from build123d import *

# Parameters (mm, degrees)
F1_DEPTH = 152.4


with BuildPart() as f1:
    # F0 (on Front) → F1 (new body)
    with BuildSketch(Plane.XZ):
        Polygon((-58.954738, 0), (0, 0), (0, 16.688244), (-43.046318, 16.688244), (-43.046318, 30.101229), (-43.046318, 54.935103), (-58.954738, 60.358422), align=None)
    extrude(amount=F1_DEPTH)

    # F1_face (on face) → F2 (revolve)
    with BuildSketch(Plane(origin=(-38.122493, -152.4, 19.839762), x_dir=(1, 0, 0), z_dir=(0, -1, 0))):
        Polygon((-20.832245, 40.51866), (-20.832245, -19.839762), (38.122493, -19.839762), (38.122493, -3.151518), (-4.923825, -3.151518), (-4.923825, 35.095341), align=None)
    revolve(axis=Axis((0, -152.4, 8.344122), (0, 0, -1)))


solid = f1.part
Work out the finished part from the listing and answer in its coordinate system (mm). A direction names the side the tool comes from. Coordinates: 2 decimals unless noted, no trailing zeros. Write each loop counter-clockwise with the first axis right and the second up, starting at its lowest first coordinate (ties: lowest second). Pieces come first, ordered by that corner, then holes.
1. For a pull along X with two mould halves and no side action, classify faces 1 (the conical face through (5.733, -108.733, 55.274)), 2 (the flat face through (-12, -128, 0)), 3 (the flat face through (0, -46, 8)) as +X half, -X half, draft (parallel to the pull), parting line (faces both ways), or undercut.
Results list:
face 1: undercut
face 2: draft
face 3: +X half
2. Flat-ended cylindrical pins translate along their axes: pin 1 (10 mm diameter, centred on x = 38, y = -172, fed in from -Z); pin 2 (10 mm diameter, centred on y = -85, z = 54, fed in from +X); pin 3 (4 mm diameter, centred on x = -12, z = 43, fed in from -Y); pin 4 (2 mm diameter, centred on x = 7.5, z = 43.5, fed in from -Y). Find the tip coordinate at first contact, or state that the pin passes through.
Results list:
pin 1: stops at z = 0
pin 2: stops at x = -43.05
pin 3: stops at y = -210.5
pin 4: stops at y = -211
3. The part is cut by section B-B, the plane y = -57. Write down the section's boundary in (x, z), and give its area (3 significant figures).
Results list:
outline: (-58.95, 0) - (0, 0) - (0, 16.69) - (-43.05, 16.69) - (-43.05, 54.94) - (-58.95, 60.36) - close
area: 1,640 mm2
4. The part is cut by section A-A, the plane z = 19. Write down the section's boundary in (x, y).
Results list:
outline: (-58.95, -152.4) arc R58.95 ccw (long way) to (-43.05, -112.12) - (-43.05, 0) - (-58.95, 0) - close; hole circle Ø86.09 at (0, -152.4)
5. For faces 4 (the flat face through (-50.89, -58.2, 57.61)), 5 (the cylindrical face through (5.6, -109.72, 36.08)), 6 (the flat face through (-58.955, -75, 31)), determine the directions among +Z, -Z, +X, -X, +Y, -Y from which every point of the face is accessible in a straight line to the end or side of a thin tool.
Results list:
face 4: +Z, +Y
face 5: +Z
face 6: +Z, -Z, -X, +Y, -Y
6. Consider line 1 along X through (y, z) = (-152, 36); line 2 along Y through (x, z) = (0, 30); line 3 along Z through (x, y) = (20, -146.5). Determine where each line is inside the solid, lowest interval first.
Results list:
line 1: x = -58.95 to -43.04, 43.04 to 58.95
line 2: y = -211.35 to -195.45, -109.35 to -93.45
line 3: z = 0 to 16.69
